Read the model definition and answer for the solid it produces. Units are mm, in the model's axes. Coordinates: 2 decimals unless noted, no trailing zeros. Order: outer loops, then holes, each group sorted by start corner. A loop starts at its lowest first (then second) coordinate and runs counter-clockwise, first axis right, second up. Notation, with made-up numbers: (-21, 47.25) - (-3, 47.25) arc R35 cw to (-3, 83.25) - close; hole circle Ø6 at (75, -21.75). An arc over 180 degrees is marked (long way). Write item = value, one per line.
from build123d import *
from OCP.BRepFilletAPI import BRepFilletAPI_MakeChamfer

# Parameters (mm, degrees)
BOSS_EXTRUDE1_DEPTH = 1.143
CHAMFER1_SIZE       = 0.635
CHAMFER1_SIZE2      = 0.366617421
SCALE1_SCALE        = 0.654


with BuildPart() as part:
    # Sketch1 → Boss-Extrude1 (new body)
    with BuildSketch(Plane(origin=(0, 0, 0), x_dir=(0, 0, -1), z_dir=(1, 0, 0))):
        with BuildLine():
            Line((8.9789, 2.286), (8.9789, 20.955))
            Line((8.9789, 20.955), (7.8359, 20.955))
            Line((7.8359, 20.955), (7.8359, 2.286))
            ThreePointArc((7.8359, 2.286), (7.501123051, 1.477776949), (6.6929, 1.143))
            Line((6.6929, 1.143), (0, 1.143))
            Line((0, 1.143), (0, 0))
            Line((0, 0), (6.6929, 0))
            ThreePointArc((6.6929, 0), (8.309346102, 0.669553898), (8.9789, 2.286))
        make_face()
    extrude(amount=BOSS_EXTRUDE1_DEPTH)

    # Chamfer1: one chamfer whose edges measure the first distance from different faces: ONE call of the kernel's chamfer builder (chamfer() names one face for all edges)
    chamfer1_edges_1 = [part.edges().sort_by_distance(p)[0] for p in [
        (0.5715, 20.955, -7.8359),
    ]]
    chamfer1_side_1 = [part.faces().sort_by_distance(p)[0] for p in [
        (0.5715, 11.6205, -7.8359),
    ]]
    chamfer1_edges_2 = [part.edges().sort_by_distance(p)[0] for p in [
        (0.5715, 20.955, -8.9789),
    ]]
    chamfer1_side_2 = [part.faces().sort_by_distance(p)[0] for p in [
        (0.5715, 11.6205, -8.9789),
    ]]
    chamfer1_edges_3 = [part.edges().sort_by_distance(p)[0] for p in [
        (1.143, 20.955, -8.4074),
    ]]
    chamfer1_side_3 = [part.faces().sort_by_distance(p)[0] for p in [
        (1.143, 0.8307576, -8.1481424),
    ]]
    chamfer1_edges_4 = [part.edges().sort_by_distance(p)[0] for p in [
        (0, 20.955, -8.4074),
    ]]
    chamfer1_side_4 = [part.faces().sort_by_distance(p)[0] for p in [
        (0, 0.8307576, -8.1481424),
    ]]
    chamfer1 = BRepFilletAPI_MakeChamfer(part.part.solid().wrapped)
    for e in chamfer1_edges_1:
        chamfer1.Add(CHAMFER1_SIZE, CHAMFER1_SIZE2, e.wrapped, chamfer1_side_1[0].wrapped)  # the first distance lies on this face
    for e in chamfer1_edges_2:
        chamfer1.Add(CHAMFER1_SIZE, CHAMFER1_SIZE2, e.wrapped, chamfer1_side_2[0].wrapped)  # the first distance lies on this face
    for e in chamfer1_edges_3:
        chamfer1.Add(CHAMFER1_SIZE, CHAMFER1_SIZE2, e.wrapped, chamfer1_side_3[0].wrapped)  # the first distance lies on this face
    for e in chamfer1_edges_4:
        chamfer1.Add(CHAMFER1_SIZE, CHAMFER1_SIZE2, e.wrapped, chamfer1_side_4[0].wrapped)  # the first distance lies on this face
    add(Compound.cast(chamfer1.Shape()), mode=Mode.REPLACE)


with BuildPart() as part_1:
    # Scale1: scaled about (0.5715, 7.832685678, -7.129530876)
    add(part.part.scale(SCALE1_SCALE).moved(Location((0.197739, 2.710109245, -2.466817683))))


solid = part_1.part
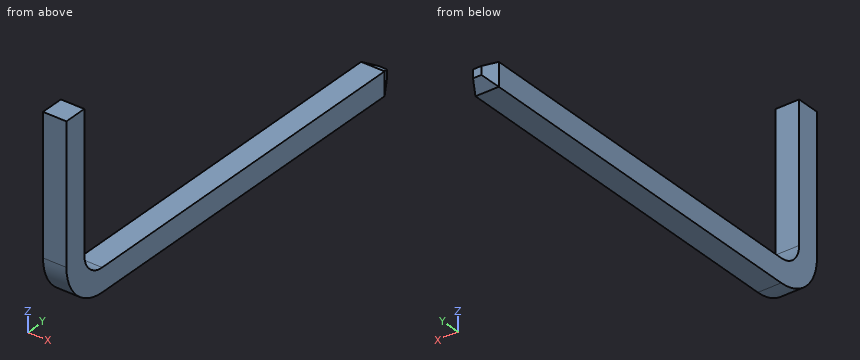
1) Straight lines are drawn through the part: line 1 along Z through (x, y) = (0.75, 5.5); line 2 along Y through (x, z) = (0.3, -5.8); line 3 along Y through (x, z) = (0.85, -8.05). For each, find the intervals that lie inside material, in ascending order. Write a range as from..to.
Returned:
line_1 = -8.34..-7.59
line_2 = 2.71..3.46
line_3 = 3.32..16.16
2) The part is cut by section A-A (x = 0.55). Determine the outline of the cut face in (y, z).
Returned:
outline = (2.71, -6.84) arc R1.5 ccw to (4.21, -8.34) - (16, -8.34) - (16.41, -8.1) - (16.41, -7.83) - (16, -7.59) - (4.21, -7.59) arc R0.75 cw to (3.46, -6.84) - (3.46, -2.47) - (2.71, -2.47) - close
3) The part is cut by section B-B (z = -5.65). Determine the outline of the cut face in (x, y).
Returned:
outline = (0.2, 2.71) - (0.95, 2.71) - (0.95, 3.46) - (0.2, 3.46) - close
4) The part is cut by section C-C (y = 14.75). Determine the outline of the cut face in (x, z).
Returned:
outline = (0.2, -8.34) - (0.95, -8.34) - (0.95, -7.59) - (0.2, -7.59) - close
